Can you work these out from the model? Positions are in its coordinate system, mm. A direction names the side the tool comes from. Coordinates: 2 decimals unless noted, no trailing zeros. Write each loop counter-clockwise with the first axis right and the second up, starting at its lowest first coordinate (ties: lowest second). Pieces come first, ordered by that corner, then holes. Notation, with made-up numbers: M -27,75.5 L -8,75.5 A15 cw -8,92.5 Z; hole C -34.5,53 d5. An arc over 180 degrees is marked long. Answer as a JSON object with one key per item and string values. Group by question number.
from build123d import *

# Parameters (mm, degrees)
F0_W      = 23.5
F0_H      = 62
F1_DEPTH  = 1.5
F2_W      = 26.5
F2_H      = 65
F2_W_2    = 23.5
F2_H_2    = 62
F3_DEPTH  = 12
F4_W      = 2
F4_H      = 39
F5_DEPTH  = 7
F7_DEPTH  = 7
F8_W      = 19
F8_H      = 5
F9_DEPTH  = 8
F11_DEPTH = 6
F12_R     = 5
F13_DEPTH = 3
F14_SIZE  = 1.49999


# Not quite as in the source:
# - a fillet or chamfer is up to 0.001 mm smaller than in the source, because OpenCascade refuses the exact size


with BuildPart() as f1:
    # F0 (on Top) → F1 (new body)
    with BuildSketch(Plane.XY):
        Rectangle(F0_W, F0_H)
    extrude(amount=F1_DEPTH)

    # F2 (on Top) → F3 (join)
    with BuildSketch(Plane.XY):
        Rectangle(F2_W, F2_H)
        Rectangle(F2_W_2, F2_H_2, mode=Mode.SUBTRACT)
    extrude(amount=F3_DEPTH)

    # F4 (on face) → F5 (join)
    with BuildSketch(Plane.XY.offset(12)):
        with Locations((-13.75, -1.5)):
            Rectangle(F4_W, F4_H)
        with Locations((13.75, -1.5)):
            Rectangle(F4_W, F4_H)
    extrude(amount=F5_DEPTH)

    # F6 (on face) → F7 (join, through all)
    with BuildSketch(Plane.XY.offset(12)):
        Polygon((14.75, -21), (11.75, -21), (11.75, -22.5), (13.25, -22.5), align=None)
        Polygon((11.75, 19.5), (11.75, 18), (14.75, 18), (13.25, 19.5), align=None)
        Polygon((-13.25, 19.5), (-14.75, 18), (-11.75, 18), (-11.75, 19.5), align=None)
        Polygon((-11.75, -22.5), (-11.75, -21), (-14.75, -21), (-13.25, -22.5), align=None)
    extrude(amount=F7_DEPTH)

    # F8 (on face) → F9 (cut)
    with BuildSketch(Plane.XY.offset(1.5)):
        with Locations((0, 31)):
            Rectangle(F8_W, F8_H)
    extrude(amount=F9_DEPTH, mode=Mode.SUBTRACT)

    # F10 (on face) → F11 (cut)
    with BuildSketch(Plane.XY.offset(12)):
        Polygon((-13.25, -25.5), (-13.25, -32.5), (-3.25, -32.5), (-3.25, -31), (-11.75, -31), (-11.75, -25.5), align=None)
    extrude(amount=-F11_DEPTH, mode=Mode.SUBTRACT)

    # F12
    f12_edges = [f1.edges().sort_by_distance(p)[0] for p in [
        (-3.25, -31.75, 6),
    ]]
    fillet(f12_edges, radius=F12_R)

    # F13 (add): faces of the model
    f13_faces = [f1.faces().sort_by_distance(p)[0] for p in [
        (-13.9907407407, -1.5, 12),
        (13.9907407407, -1.5, 12),
    ]]
    extrude(f13_faces, amount=F13_DEPTH)

    # F14 (size 1.5 in the source; OpenCascade refuses exactly that, so slightly less here)
    f14_edges = [f1.edges().sort_by_distance(p)[0] for p in [
        (-14.75, -1.5, 9),
        (14.75, -1.5, 9),
    ]]
    chamfer(f14_edges, length=F14_SIZE)


solid = f1.part
Q1. We'd pull the mould along Z, two halves only. Please class faces 1 (the flat face through (-9.5, 32, 5)), 2 (the flat face through (-11.75, 0, 6)), 3 (the flat face through (14, -1, 19)): pulls with the +Z half, pulls with the -Z half, needs draft (parallel to the pull), parting line crosses it, or undercut.
Q2. Please list where these lines run through material, in increasing order: L1, parallel to Y at x = -11.25, z = 5.5; L2, parallel to X at y = -15.5, z = 3.75; L3, parallel to X at y = -8, z = 10.75.
Q3. If we section it at A-A on x = 8.75: List the corners of the cut face in (y, z) for me, and give its area (3 significant figures).
Q4. Will these pins go through, and if not, where does the flat tip stop? pin 1 (3 mm diameter, centred on y = 23, z = 9, fed in from +X); pin 2 (10 mm diameter, centred on y = 9.5, z = 6, fed in from +X); pin 3 (0.5 mm diameter, centred on y = -31.5, z = 11.5, fed in from -X); pin 4 (1.2 mm diameter, centred on x = -12, z = 8, fed in from -Y).
Q5. If we section it at D-D on z = 3.5: List the corners of the cut face in (x, y) for me.
Q6. If we section it at B-B on z = 16.25: List the corners of the cut face in (x, y) for me, and give its area (4 significant figures).
Q7. On a 3-axis mill with a long thin cutter (end or side, diameter ignored), from which of +Z, -Z, +X, -X, +Y, -Y can I reach the whole of each face in a straight line? I mean faces 4 (the flat face through (-12.75, -2, 15)), 5 (the flat face through (-12, 19.5, 15)), 6 (the flat face through (9.5, 32, 5)), 7 (the flat face through (-13, -24, 12)). Say none if no direction works.
Reply:
{
 "1": {"face 1": "undercut", "face 2": "needs draft", "face 3": "pulls with the +Z half"},
 "2": {"L1": "-32.5 to -31, 31 to 32.5", "L2": "-13.25 to -11.75, 11.75 to 13.25", "L3": "-14.75 to -11.75, 11.75 to 14.75"},
 "3": {"outline": "M -32.5,0 L 32.5,0 L 32.5,1.5 L -31,1.5 L -31,12 L -32.5,12 Z; M 31,9.5 L 32.5,9.5 L 32.5,12 L 31,12 Z", "area": "117 mm^2"},
 "4": {"pin 1": "x = 13.25", "pin 2": "x = 14.75", "pin 3": "x = -3.25", "pin 4": "y = -25.5"},
 "5": {"outline": "M -13.25,-32.5 L 13.25,-32.5 L 13.25,32.5 L 9.5,32.5 L 9.5,31 L 11.75,31 L 11.75,-31 L -11.75,-31 L -11.75,31 L -9.5,31 L -9.5,32.5 L -13.25,32.5 Z"},
 "6": {"outline": "M -14.75,-21 L -13.25,-22.5 L -11.75,-22.5 L -11.75,-21 L -12.75,-21 L -12.75,18 L -11.75,18 L -11.75,19.5 L -13.25,19.5 L -14.75,18 Z; M 11.75,-22.5 L 13.25,-22.5 L 14.75,-21 L 14.75,18 L 13.25,19.5 L 11.75,19.5 L 11.75,18 L 12.75,18 L 12.75,-21 L 11.75,-21 Z", "area": "169.5 mm^2"},
 "7": {"face 4": "+Z", "face 5": "+Z, +X, -X, +Y", "face 6": "+Y", "face 7": "+Z, +X, -X, -Y"}
}
